The listing builds one solid part. Answer for the finished solid, in the listing's coordinates (mm). A direction names the side the tool comes from. Coordinates: 2 decimals unless noted, no trailing zeros. Write each loop counter-clockwise with the first axis right and the second up, starting at its lowest first coordinate (ties: lowest second). Pieces come first, ordered by that corner, then holes.
from build123d import *

# Parameters (mm, degrees)
SKETCH1_R           = 90
BOSS_EXTRUDE1_DEPTH = 16
SKETCH2_R           = 5
CUT_EXTRUDE1_DEPTH  = 129.280941687
SKETCH3_R           = 6.513808384
CUT_EXTRUDE2_DEPTH  = 10.201452
CIRPATTERN1_START   = 5.798548075
CIRPATTERN1_DEPTH   = 10.201451925


# Read off the part's stored shape, not the designer's step: CirPattern1
with BuildPart() as part:
    # Sketch1 → Boss-Extrude1 (new body)
    with BuildSketch(Plane(origin=(0, 0, 0), x_dir=(1, 0, 0), z_dir=(0, 1, 0))):
        with Locations(Location((0, 0, 0), (0, 0, 270))):
            Circle(SKETCH1_R)
    extrude(amount=BOSS_EXTRUDE1_DEPTH)

    # Sketch2 → Cut-Extrude1 (cut, through all)
    with BuildSketch(Plane(origin=(0, 0, 0), x_dir=(1, 0, 0), z_dir=(0, 1, 0))):
        with Locations(Location((0, 0, 0), (0, 0, 270))):
            Circle(SKETCH2_R)
    extrude(amount=CUT_EXTRUDE1_DEPTH, mode=Mode.SUBTRACT)

    # Sketch3 → Cut-Extrude2 (cut)
    with BuildSketch(Plane(origin=(0, 16, 0), x_dir=(1, 0, 0), z_dir=(0, 1, 0))):
        with Locations((-7.214525681, 0)):
            Circle(SKETCH3_R)
    extrude(amount=-CUT_EXTRUDE2_DEPTH, mode=Mode.SUBTRACT)

    # CirPattern1 outline → CirPattern1 (cut)
    with BuildSketch(Plane(origin=(0, 0, 0), x_dir=(1, 0, 0), z_dir=(0, 1, 0)).offset(CIRPATTERN1_START)):
        with BuildLine():
            ThreePointArc((-2.399304034, -4.386723168), (-2.558979696, -4.555830467), (-2.724590711, -4.719129542))
            ThreePointArc((-2.724590711, -4.719129542), (6.864167033, -11.889086052), (5.449181423, 0))
            ThreePointArc((5.449181423, 0), (6.864167033, 11.889086052), (-2.724590711, 4.719129542))
            ThreePointArc((-2.724590711, 4.719129542), (-2.558979696, 4.555830467), (-2.399304034, 4.386723168))
            ThreePointArc((-2.399304034, 4.386723168), (5, 0), (-2.399304034, -4.386723168))
        make_face()
    extrude(amount=CIRPATTERN1_DEPTH, mode=Mode.SUBTRACT)


solid = part.part
1. Section B-B on z = -29.5 is taken. Give the vertices of the cut face in (x, y).
Results found:
outline: (-85.03, 0) - (85.03, 0) - (85.03, 16) - (-85.03, 16) - close
2. For a pull along Z with two mould halves and no side action, classify faces 3 (the flat face through (-19, 0, -1)), 4 (the cylindrical face through (-34.471, 7.888, 83.137)), 5 (the cylindrical face through (6.68, 10.83, 11.99)) as pulls with the +Z half, pulls with the -Z half, needs draft (parallel to the pull), parting line crosses it, or undercut.
Results found:
face 3: needs draft
face 4: parting line crosses it
face 5: undercut
3. Flat-ended cylindrical pins translate along their axes: P1, Ø5, axis at x = -43.5, y = 2.5, coming from the -Z side; P2, Ø6, axis at y = 4, z = -70.5, coming from the -X side; P3, Ø3, axis at x = 64, y = 5.5, coming from the +Z side. Find the tip coordinate at first contact, or state that the pin passes through.
Results found:
P1: stops at z = -80.12
P2: stops at x = -59.53
P3: stops at z = 64.76
4. Section A-A on x = 0 is taken. Give the vertices of the cut face in (y, z).
Results found:
outline: (0, -90) - (16, -90) - (16, -11.67) - (5.8, -11.67) - (5.8, -5) - (0, -5) - close; (0, 5) - (5.8, 5) - (5.8, 11.67) - (16, 11.67) - (16, 90) - (0, 90) - close
5. Section D-D on y = 13.25 is taken. Give the vertices of the cut face in (x, z).
Results found:
outline: circle Ø180 at (0, 0); hole (-2.72, -4.72) arc R6.51 ccw (long way) to (5.45, 0) arc R6.51 ccw (long way) to (-2.72, 4.72) arc R6.51 ccw (long way) to start
6. A tool of negligible diameter and unlimited length cuts with its end or side. For faces 1 (the flat face through (-19, 16, -1)), 2 (the cylindrical face through (7.047, 10.828, -11.78)), from which of +Z, -Z, +X, -X, +Y, -Y can it reach the whole face along a straight path? Write none if from no direction.
Results found:
face 1: +Z, -Z, +X, -X, +Y
face 2: +Y
7. Section C-C on x = -49 is taken. Give the vertices of the cut face in (y, z).
Results found:
outline: (0, -75.49) - (16, -75.49) - (16, 75.49) - (0, 75.49) - close
8. Find the intervals of material crossed by L1, parallel to X at y = 1.25, z = 0; L2, parallel to Z at x = -12, y = 13.75; L3, parallel to Z at x = -2.5, y = 3.5, in increasing order.
Results found:
L1: x = -90 to -5, 5 to 90
L2: z = -89.2 to -4.42, 4.42 to 89.2
L3: z = -89.97 to -4.33, 4.33 to 89.97
